Here's how the part is built. I have some questions about the finished solid (model axes, mm). A direction names the side the tool comes from. Round coordinates to 2 decimals unless told otherwise and drop trailing zeros. Loops run counter-clockwise (first coordinate to the right, second up) from the corner with the lowest first, then second, coordinate; pieces in that order, holes last. Notation, with made-up numbers: M 88.5,53.5 L 106.5,53.5 A24 ccw 106.5,68.5 Z; hole C 69,-12 d6. An arc over 180 degrees is marked long. Answer as a JSON object with one key per item and string values.
from build123d import *

# Parameters (mm, degrees)
SKIZZE2_R                       = 7.5
SKIZZE2_R_2                     = 3
AUFSATZ_LINEAR_AUSTRAGEN1_DEPTH = 10


with BuildPart() as part:
    # Skizze1 → Rotation1 (revolve)
    with BuildSketch(Plane(origin=(0, 0, 0), x_dir=(0, 0, -1), z_dir=(1, 0, 0))):
        Polygon((-3, 0), (-27.5, 0), (-27.5, -5), (-7.5, -5), (-7.5, -32), (-3, -32), align=None)
    revolve(axis=Axis((0, 21.68541583, 0), (0, -1, 0)))

    # Skizze2 → Aufsatz-Linear austragen1 (add)
    with BuildSketch(Plane(origin=(0, 0, 0), x_dir=(1, 0, 0), z_dir=(0, 1, 0))):
        Circle(SKIZZE2_R)
        Circle(SKIZZE2_R_2, mode=Mode.SUBTRACT)
    extrude(amount=AUFSATZ_LINEAR_AUSTRAGEN1_DEPTH)


solid = part.part
Item 1: I want a section at B-B on z = 0. List the corners of the cut face in (x, y) for me, plus the area to 3 significant figures.
Solution:
{"outline": "M -27.5,-5 L -7.5,-5 L -7.5,-32 L -3,-32 L -3,10 L -7.5,10 L -7.5,0 L -27.5,0 Z; M 3,-32 L 7.5,-32 L 7.5,-5 L 27.5,-5 L 27.5,0 L 7.5,0 L 7.5,10 L 3,10 Z", "area": "578 mm2"}
Item 2: For faces 1 (the face through (6, 0, -6)), 2 (the face through (-0.33, -18.689, -7.493)), 3 (the face through (3.2, 10, -0.1)), which set-ups out of +Z, -Z, +X, -X, +Y, -Y let a thin tool reach every point of the face, with its end or its side?
Solution:
{"face 1": "+Y", "face 2": "-Y", "face 3": "+Z, -Z, +X, -X, +Y"}
Item 3: For P1, Ø3, axis at x = 15, z = -3.5, coming from the +Y side; P2, Ø6, axis at x = 12.5, z = 7.5, coming from the -Y side; P3, Ø5, axis at y = -7, z = -20.5, coming from the +X side, each with a flat end and sliding along its axis, tell me the tip position at first contact or that it passes through.
Solution:
{"P1": "stops at y = 0", "P2": "stops at y = -5", "P3": "stops at x = 19.88"}
Item 4: I want a section at C-C on y = -18. List the corners of the cut face in (x, z) for me.
Solution:
{"outline": "C 0,0 d15; hole C 0,0 d6"}
Item 5: If I drill on L1, parallel to X at y = -25, z = 0; L2, parallel to Y at x = -17, z = 9.5, over which ranges is the centre line in solid material (lowest first)? Write a range as from..to.
Solution:
{"L1": "x = -7.5..-3, 3..7.5", "L2": "y = -5..0"}
Item 6: I want a section at A-A on x = 0. List the corners of the cut face in (y, z) for me.
Solution:
{"outline": "M -32,-7.5 L -5,-7.5 L -5,-27.5 L 0,-27.5 L 0,-7.5 L 10,-7.5 L 10,-3 L -32,-3 Z; M -32,3 L 10,3 L 10,7.5 L 0,7.5 L 0,27.5 L -5,27.5 L -5,7.5 L -32,7.5 Z"}
Item 7: I want a section at D-D on z = 6.5. List the corners of the cut face in (x, y) for me.
Solution:
{"outline": "M -26.72,-5 L -3.74,-5 L -3.74,-32 L 3.74,-32 L 3.74,-5 L 26.72,-5 L 26.72,0 L 3.74,0 L 3.74,10 L -3.74,10 L -3.74,0 L -26.72,0 Z"}
